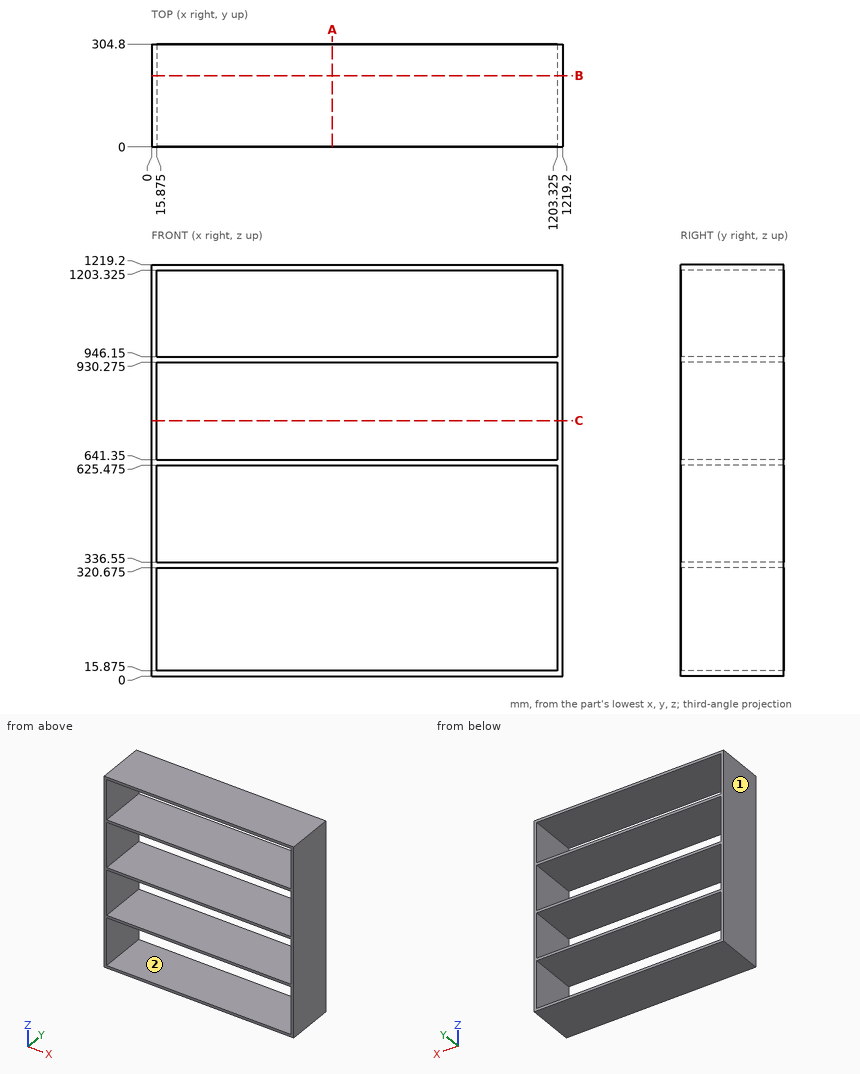
Source: three-view drawing plus pictorial views. Frame: mm from the lowest corner of the part. A direction names the side the tool comes from. Round coordinates to 2 decimals unless told otherwise and drop trailing zeros. Loops run counter-clockwise (first coordinate to the right, second up) from the corner with the lowest first, then second, coordinate; pieces in that order, holes last. Notation, with made-up numbers: M -17.75,76 L -3.75,76 A6 cw -3.75,87 Z; hole C -5.75,88 d4. An arc over 180 degrees is marked long. Put each result on its own line as item: value. Start each with the question number.
(1) Section query C-C (z = 757). Return loops of the section in (x, y) (3 decimals).
(2) Set-up query: the marked faces 1 and 2. Return all of +Z, -Z, +X, -X, +Y, -Y with unobstructed straight access to the full face (end or side cutting, diameter ignored); none if empty.
(3) Section query A-A (x = 536.5). Return loops of the section in (y, z) (3 decimals).
(4) Section query B-B (y = 211). Return loops of the section in (x, z) (3 decimals).
(5) Material intervals for line 1 along Z through (x, y) = (796, 232.5) (3 decimals); line 2 along X through (y, z) = (220, 877) (3 decimals), sorted ascending. Write a range as [from, to].
Findings below:
1. outline: M 0,0 L 15.875,0 L 15.875,304.8 L 0,304.8 Z; M 1203.325,0 L 1219.2,0 L 1219.2,304.8 L 1203.325,304.8 Z
2. face 1: +Z, -Z, -X, +Y, -Y
2. face 2: +Y, -Y
3. outline: M 0,0 L 304.8,0 L 304.8,15.875 L 0,15.875 Z; M 0,320.675 L 304.8,320.675 L 304.8,336.55 L 0,336.55 Z; M 0,625.475 L 304.8,625.475 L 304.8,641.35 L 0,641.35 Z; M 0,930.275 L 304.8,930.275 L 304.8,946.15 L 0,946.15 Z; M 0,1203.325 L 304.8,1203.325 L 304.8,1219.2 L 0,1219.2 Z
4. outline: M 0,0 L 1219.2,0 L 1219.2,1219.2 L 0,1219.2 Z; hole M 15.875,15.875 L 1203.325,15.875 L 1203.325,320.675 L 15.875,320.675 Z; hole M 15.875,336.55 L 1203.325,336.55 L 1203.325,625.475 L 15.875,625.475 Z; hole M 15.875,641.35 L 1203.325,641.35 L 1203.325,930.275 L 15.875,930.275 Z; hole M 15.875,946.15 L 1203.325,946.15 L 1203.325,1203.325 L 15.875,1203.325 Z
5. line 1: z = [0, 15.875], [320.675, 336.55], [625.475, 641.35], [930.275, 946.15], [1203.325, 1219.2]
5. line 2: x = [0, 15.875], [1203.325, 1219.2]
